Geometry: final body of the model. Coordinates: model frame, mm. Face numbers are marked on the shaded views. A direction names the side the tool comes from. Give positions to 0.01 mm unless a question says otherwise; leave off trailing zeros. Write each loop counter-clockwise with the first axis right and the second up, starting at its lowest first coordinate (ties: lowest second). Pieces come first, ordered by that corner, then holes. Notation, with made-up numbers: M 80,40.5 L 122,40.5 A15 ccw 122,45.5 Z; hole C 83.25,7.25 d5. An arc over 180 degrees is marked long. Use a Markdown table: item, result. Add a question column.
1) Set-up query: the marked faces 1, 2 and 3. Return all of +Z, -Z, +X, -X, +Y, -Y with unobstructed straight access to the full face (end or side cutting, diameter ignored); none if empty.
2) Section C-C on z = 48. State how many separate pieces and enclosed holes the cut face has, then the cut area to 3 significant figures.
3) Section B-B on y = 16. Return the cut outline in (x, z), then the cut area to 3 significant figures.
4) Draft query along Y for the marked faces 4, 5 and 6. Return one class per face: +Y half, -Y half, draft (parallel to the pull), parting line (faces both ways), or undercut.
5) Section A-A on x = 34.5. Return the cut outline in (y, z).
6) Line query: line 1 (Y direction, x = 30.5, z = 47); line 2 (X direction, y = 18, z = 37); line 3 (X direction, y = 42, z = 42). Output: solid intervals per line, ascending.
7) Section D-D on y = 9.5. Return the cut outline in (x, z).
8) Pin query (flat end, axial travel): pin 1 (8.5 mm diameter, centred on x = 47.12, z = 46.77, fed in from -Y); pin 2 (12 mm diameter, centred on y = 38.5, z = 50, fed in from +X); pin 3 (17.5 mm diameter, centred on x = 47, z = 38, fed in from -Y); pin 4 (8.5 mm diameter, centred on y = 39.89, z = 46.77, fed in from +X). Return the tip coordinate at first contact, or that it passes through.
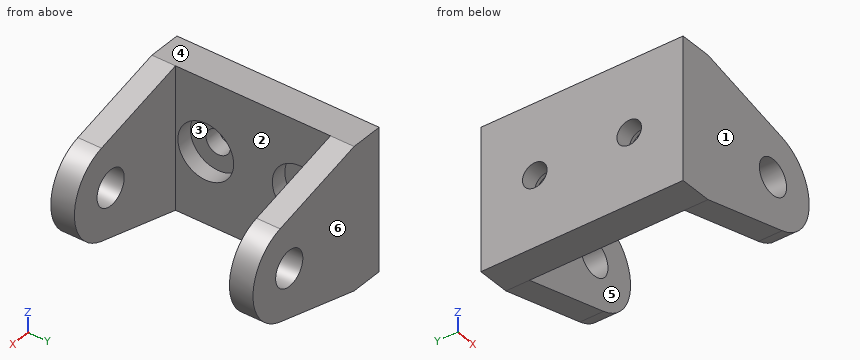
```python
from build123d import *

# Parameters (mm, degrees)
SKETCH1_W                               = 8.76
SKETCH1_H                               = 38.1
BOSS_EXTRUDE1_DEPTH                     = 54.37886
CBORE_FOR_M6_HEX_HEAD_BOLT1_D           = 6.6
CBORE_FOR_M6_HEX_HEAD_BOLT1_DEPTH       = 14.019159957
CBORE_FOR_M6_HEX_HEAD_BOLT1_CBORE_D     = 15
CBORE_FOR_M6_HEX_HEAD_BOLT1_CBORE_DEPTH = 4.38
CBORE_FOR_M6_HEX_HEAD_BOLT1_TIP         = 1.982840043
SKETCH6_R                               = 4.7625
BOSS_EXTRUDE2_DEPTH                     = 6.35


with BuildPart() as part:
    # Sketch1 → Boss-Extrude1 (new body)
    with BuildSketch(Plane(origin=(0, 0, 0), x_dir=(1, 0, 0), z_dir=(0, 1, 0))):
        with Locations((20.010864679, -46.77095316)):
            Rectangle(SKETCH1_W, SKETCH1_H)
    extrude(amount=BOSS_EXTRUDE1_DEPTH)

    # CBORE for M6 Hex Head Bolt1
    with Locations(Plane(origin=(24.390864679, 0, 0), x_dir=(0, 0, -1), z_dir=(1, 0, 0))):
        with Locations((-46.77095316, 14.48943), (-46.77095316, 39.88943)):
            CounterBoreHole(CBORE_FOR_M6_HEX_HEAD_BOLT1_D / 2, CBORE_FOR_M6_HEX_HEAD_BOLT1_CBORE_D / 2, CBORE_FOR_M6_HEX_HEAD_BOLT1_CBORE_DEPTH, depth=CBORE_FOR_M6_HEX_HEAD_BOLT1_DEPTH)
            with Locations((0, 0, -(CBORE_FOR_M6_HEX_HEAD_BOLT1_DEPTH + CBORE_FOR_M6_HEX_HEAD_BOLT1_TIP / 2))):  # 118° drill point
                Cone(0, CBORE_FOR_M6_HEX_HEAD_BOLT1_D / 2, CBORE_FOR_M6_HEX_HEAD_BOLT1_TIP, mode=Mode.SUBTRACT)

    # Sketch6 → Boss-Extrude2 (add)
    with BuildSketch(Plane(origin=(0, 54.37886, 0), x_dir=(1, 0, 0), z_dir=(0, 1, 0))):
        with BuildLine():
            Line((24.390864679, -27.72095316), (24.390864679, -65.82095316))
            Line((24.390864679, -65.82095316), (50.322824333, -59.060163405))
            ThreePointArc((50.322824333, -59.060163405), (59.818871843, -46.77095316), (50.322824333, -34.481742916))
            Line((50.322824333, -34.481742916), (24.390864679, -27.72095316))
        make_face()
        with Locations(Location((47.118871843, -46.77095316, 0), (0, 0, 270))):
            Circle(SKETCH6_R, mode=Mode.SUBTRACT)
    boss_extrude2 = extrude(amount=-BOSS_EXTRUDE2_DEPTH)

    # Mirror1: Boss-Extrude2 across plane
    add(boss_extrude2.mirror(Plane.ZX.offset(27.18943)))


solid = part.part
```
Found:
| question | item | result |
|---|---|---|
| 1 | face 1 | +Z, -Z, +X, -X, -Y |
| 1 | face 2 | +Z, -Z, +X |
| 1 | face 3 | +X |
| 2 | separate pieces | 5 |
| 2 | enclosed holes | 0 |
| 2 | area | 625 mm² |
| 3 | outline | M 15.63,27.72 L 24.39,27.72 L 24.39,39.42 L 20.01,39.42 L 20.01,43.84 L 15.63,43.84 Z; M 15.63,49.7 L 20.01,49.7 L 20.01,54.12 L 24.39,54.12 L 24.39,65.82 L 15.63,65.82 Z |
| 3 | area | 244 mm² |
| 4 | face 4 | draft |
| 4 | face 5 | undercut |
| 4 | face 6 | +Y half |
| 5 | outline | M 0,30.36 L 6.35,30.36 L 6.35,63.19 L 0,63.19 Z; M 48.03,30.36 L 54.38,30.36 L 54.38,63.19 L 48.03,63.19 Z |
| 6 | line 1 | 0 to 6.35, 48.03 to 54.38 |
| 6 | line 2 | 15.63 to 24.39 |
| 6 | line 3 | 15.63 to 20.01 |
| 7 | outline | M 15.63,27.72 L 24.39,27.72 L 24.39,41.17 L 20.01,41.17 L 20.01,52.37 L 24.39,52.37 L 24.39,65.82 L 15.63,65.82 Z |
| 8 | pin 1 | through |
| 8 | pin 2 | x = 24.39 |
| 8 | pin 3 | y = 0 |
| 8 | pin 4 | x = 20.01 |
